Source: CAD feature listing. Evaluate the final solid. Frame: model axes, mm. Face numbers are marked on the shaded views. A direction names the side the tool comes from. Give positions to 0.01 mm unless a question says otherwise; leave off trailing zeros. Write each loop counter-clockwise with the first axis right and the second up, starting at its lowest first coordinate (ties: lowest second). Pieces come first, ordered by that corner, then holes. Notation, with made-up numbers: (-8, -40) -> (4, -40) arc R6 ccw to (4, -30) -> close; hole circle Ø5 at (-26.75, -30). An arc over 180 degrees is marked (long way). Answer as a JSON object with one key per item and string values. Group by question number.
Item 1: Section query A-A on x = 1235. Return the cut outline in (y, z), plus the area to 3 significant figures.
Item 2: Ray query, probe 1 along X at (y, z) = (18.5, -79); probe 2 along Z at (x, y) = (1306.5, 54). Return the intervals inside material, ascending. Write a range as from..to.
Item 3: Access query for the marked faces 1, 2 and 3. Directions: +Z, -Z, +X, -X, +Y, -Y. A direction counts if a zero-diameter tool reaches every point of the face in a straight line with its end or side. Return the directions, or none.
Item 4: First-contact query: pin 1 Ø8 at (x, y) = (817, -72) entering from -Z; pin 2 Ø14.5 at (x, z) = (87.5, -88) entering from -Y (3 decimals); pin 3 Ø1.5 at (y, z) = (0.5, -69) entering from -X; pin 4 Ø16 at (y, z) = (3, -83.5) entering from -X. Flat tips, straight axial feed; report the tip coordinate or a pass-through.
from build123d import *

# Parameters (mm, degrees)
SKETCH3_W                = 151
SKETCH3_H                = 151
BOSS_EXTRUDE2_DEPTH      = 1724.45
SKETCH4_R                = 113.5
BOSS_EXTRUDE3_DEPTH      = 13
SKETCH5_R                = 6.74624
CUT_EXTRUDE1_DEPTH       = 13
CIRPATTERN1_COUNT        = 4
FILLET1_R                = 20
SKETCH6_W                = 80
SKETCH6_H                = 69.85
BOSS_EXTRUDE4_DEPTH      = 20
CHAMFER1_SIZE            = 13
FILLET2_R                = 2
CHAMFER1_OF_MIRROR1_SIZE = 13
SHELL1_START             = -13
SHELL1_DEPTH             = 1732.45
SHELL1_START_2           = 61.471067812
SHELL1_2_OUTLINE_W       = 59.85
SHELL1_2_OUTLINE_H       = 20
SHELL1_2_DEPTH           = 59.928932188
SHELL1_3_DEPTH           = 8
SHELL1_START_3           = -29.925
SHELL1_4_DEPTH           = 59.85


with BuildPart() as part:
    # Sketch3 → Boss-Extrude2 (new body)
    with BuildSketch(Plane(origin=(0, 0, 0), x_dir=(0, 0, -1), z_dir=(1, 0, 0))):
        Rectangle(SKETCH3_W, SKETCH3_H)
    extrude(amount=BOSS_EXTRUDE2_DEPTH)

    # Sketch4 → Boss-Extrude3 (add)
    with BuildSketch(Plane.ZY):
        with Locations(Location((0, 0, 0), (0, 0, 180))):
            Circle(SKETCH4_R)
    extrude(amount=BOSS_EXTRUDE3_DEPTH)

    # Sketch5 → Cut-Extrude1 (cut)
    with BuildSketch(Plane(origin=(0, 0, 0), x_dir=(0, 0, -1), z_dir=(1, 0, 0))):
        with Locations((100.5, 0)):
            Circle(SKETCH5_R)
    cut_extrude1 = extrude(amount=-CUT_EXTRUDE1_DEPTH, mode=Mode.SUBTRACT)

    # CirPattern1: Cut-Extrude1 ×4 about axis
    cirpattern1_axis = Axis((0, 0, 0), (1, 0, 0))
    for i in range(1, CIRPATTERN1_COUNT):
        add(cut_extrude1.rotate(cirpattern1_axis, i * 360 / CIRPATTERN1_COUNT), mode=Mode.SUBTRACT)

    # Fillet1
    fillet1_edges = [part.edges().sort_by_distance(p)[0] for p in [
        (862.225, -75.5, -75.5),
        (862.225, -75.5, 75.5),
        (862.225, 75.5, 75.5),
        (862.225, 75.5, -75.5),
    ]]
    fillet(fillet1_edges, radius=FILLET1_R)

    # Sketch6 → Boss-Extrude4 (add)
    with BuildSketch(Plane(origin=(0, 0, -75.5), x_dir=(-1, 0, 0), z_dir=(0, 0, -1))):
        with Locations((-86.4, 0)):
            Rectangle(SKETCH6_W, SKETCH6_H)
    boss_extrude4 = extrude(amount=BOSS_EXTRUDE4_DEPTH)

    # Chamfer1
    chamfer1_edges = [part.edges().sort_by_distance(p)[0] for p in [
        (46.4, 0, -95.5),
    ]]
    chamfer(chamfer1_edges, length=CHAMFER1_SIZE)

    # Fillet2
    fillet2_edges = [part.edges().sort_by_distance(p)[0] for p in [
        (92.9, -34.925, -95.5),
        (92.9, 34.925, -95.5),
    ]]
    fillet(fillet2_edges, radius=FILLET2_R)

    # Mirror1: Boss-Extrude4 across plane
    add(boss_extrude4.mirror(Plane.XY))

    # Chamfer1 of Mirror1
    chamfer1_of_mirror1_edges = [part.edges().sort_by_distance(p)[0] for p in [
        (46.4, 0, 95.5),
    ]]
    chamfer(chamfer1_of_mirror1_edges, length=CHAMFER1_OF_MIRROR1_SIZE)

    # Shell1: read off the stored shape, not the designer's step
    # Shell1 outline → Shell1 (cut)
    with BuildSketch(Plane.YZ.offset(SHELL1_START)):
        with BuildLine():
            Line((55.5, 70.5), (-55.5, 70.5))
            ThreePointArc((-55.5, 70.5), (-66.106601718, 66.106601718), (-70.5, 55.5))
            Line((-70.5, 55.5), (-70.5, -55.5))
            ThreePointArc((-70.5, -55.5), (-66.106601718, -66.106601718), (-55.5, -70.5))
            Line((-55.5, -70.5), (55.5, -70.5))
            ThreePointArc((55.5, -70.5), (66.106601718, -66.106601718), (70.5, -55.5))
            Line((70.5, -55.5), (70.5, 55.5))
            ThreePointArc((70.5, 55.5), (66.106601718, 66.106601718), (55.5, 70.5))
        make_face()
    extrude(amount=SHELL1_DEPTH, mode=Mode.SUBTRACT)

    # Shell1 2 outline → Shell1 2 (cut)
    with BuildSketch(Plane.YZ.offset(SHELL1_START_2)):
        with Locations((0, 80.5)):
            Rectangle(SHELL1_2_OUTLINE_W, SHELL1_2_OUTLINE_H)
        with Locations((0, -80.5)):
            Rectangle(SHELL1_2_OUTLINE_W, SHELL1_2_OUTLINE_H)
    extrude(amount=SHELL1_2_DEPTH, mode=Mode.SUBTRACT)

    # Shell1 3 outline → Shell1 3 (cut)
    with BuildSketch(Plane.YZ.offset(SHELL1_START)):
        with BuildLine():
            ThreePointArc((108.131969382, -8.929008763), (88.75376, 0), (108.131969382, 8.929008763))
            ThreePointArc((108.131969382, 8.929008763), (76.721085759, 76.721085759), (8.929008763, 108.131969382))
            ThreePointArc((8.929008763, 108.131969382), (0, 88.75376), (-8.929008763, 108.131969382))
            ThreePointArc((-8.929008763, 108.131969382), (-76.721085759, 76.721085759), (-108.131969382, 8.929008763))
            ThreePointArc((-108.131969382, 8.929008763), (-88.75376, 0), (-108.131969382, -8.929008763))
            ThreePointArc((-108.131969382, -8.929008763), (-76.721085759, -76.721085759), (-8.929008763, -108.131969382))
            ThreePointArc((-8.929008763, -108.131969382), (0, -88.75376), (8.929008763, -108.131969382))
            ThreePointArc((8.929008763, -108.131969382), (76.721085759, -76.721085759), (108.131969382, -8.929008763))
        make_face()
        with BuildLine():
            Line((55.5, -70.5), (-55.5, -70.5))
            ThreePointArc((-55.5, -70.5), (-66.106601718, -66.106601718), (-70.5, -55.5))
            Line((-70.5, -55.5), (-70.5, 55.5))
            ThreePointArc((-70.5, 55.5), (-66.106601718, 66.106601718), (-55.5, 70.5))
            Line((-55.5, 70.5), (55.5, 70.5))
            ThreePointArc((55.5, 70.5), (66.106601718, 66.106601718), (70.5, 55.5))
            Line((70.5, 55.5), (70.5, -55.5))
            ThreePointArc((70.5, -55.5), (66.106601718, -66.106601718), (55.5, -70.5))
        make_face(mode=Mode.SUBTRACT)
    extrude(amount=SHELL1_3_DEPTH, mode=Mode.SUBTRACT)

    # Shell1 4 outline → Shell1 4 (cut)
    with BuildSketch(Plane(origin=(0, 0, 0), x_dir=(1, 0, 0), z_dir=(0, 1, 0)).offset(SHELL1_START_3)):
        Polygon((51.4, 80.428932188), (51.4, 70.5), (61.471067812, 70.5), (61.471067812, 90.5), align=None)
        Polygon((61.471067812, -70.5), (51.4, -70.5), (51.4, -80.428932188), (61.471067812, -90.5), align=None)
    extrude(amount=SHELL1_4_DEPTH, mode=Mode.SUBTRACT)


solid = part.part
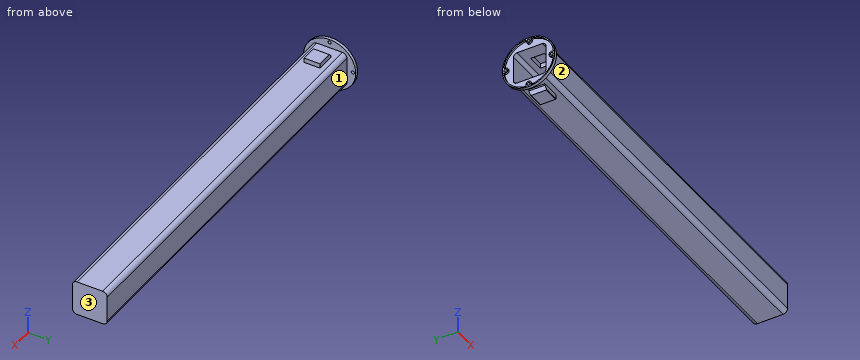
Worked answers:
{
 "1": {"outline": "(-75.5, -55.5) arc R20 ccw to (-55.5, -75.5) -> (55.5, -75.5) arc R20 ccw to (75.5, -55.5) -> (75.5, 55.5) arc R20 ccw to (55.5, 75.5) -> (-55.5, 75.5) arc R20 ccw to (-75.5, 55.5) -> close; hole (-70.5, -55.5) arc R15 ccw to (-55.5, -70.5) -> (55.5, -70.5) arc R15 ccw to (70.5, -55.5) -> (70.5, 55.5) arc R15 ccw to (55.5, 70.5) -> (-55.5, 70.5) arc R15 ccw to (-70.5, 55.5) -> close", "area": "2,770 mm^2"},
 "2": {"probe 1": "-5..0, 46.4..51.4, 121.4..126.4", "probe 2": "-75.5..-70.5, 70.5..75.5"},
 "3": {"face 1": "+Z, -Z, +X, +Y", "face 2": "+Z, -Z, +X, -Y", "face 3": "+Z, -Z, +X, +Y, -Y"},
 "4": {"pin 1": "z = -71.11", "pin 2": "y = -34.925", "pin 3": "x = 1719.45", "pin 4": "x = -13"}
}
